The drawing under review shows one solid part. Ordinate dimensions are in mm from its lowest x, y, z. A direction names the side the tool comes from. Coordinates: 2 decimals unless noted, no trailing zeros. Write each loop counter-clockwise with the first axis right and the second up, starting at its lowest first coordinate (ties: lowest second). Pieces come first, ordered by that corner, then holes.
Q1. Take a section at C-C (z = 500). Give the boundary of the cut face in (x, y).
Q2. Insertion check: pin 1 (23 mm diameter, centred on x = 50, z = 500, fed in from +Y); pin 2 (1 mm diameter, centred on x = 314, y = 10.5, fed in from -Z); pin 3 (8 mm diameter, centred on y = 23.5, z = 164.5, fed in from -X); pin 4 (8 mm diameter, centred on y = 23.5, z = 101, fed in from +X). Each pin has a flat end and moves straight along its axis. Give the tip position at first contact, or say it passes through.
Q3. Machinability: for the marked faces 1 and 2, which of the approach directions +Z, -Z, +X, -X, +Y, -Y give a long, thin tool a straight path to every point of the face, cutting with its end or side? Answer none if there is none.
Q4. Take a section at D-D (x = 250). Give the boundary of the cut face in (y, z).
Q5. For probe 1 along X at (y, z) = (10.5, 500); probe 2 along Z at (x, y) = (450, 14.5); probe 3 along X at (y, z) = (27.5, 50), list the stretches that pass through material, from the lowest coordinate up.
Q6. Take a section at A-A (x = 450). Give the boundary of the cut face in (y, z), and give its area (3 significant figures).
Q7. Take a section at B-B (y = 24.5). Give the boundary of the cut face in (x, z).
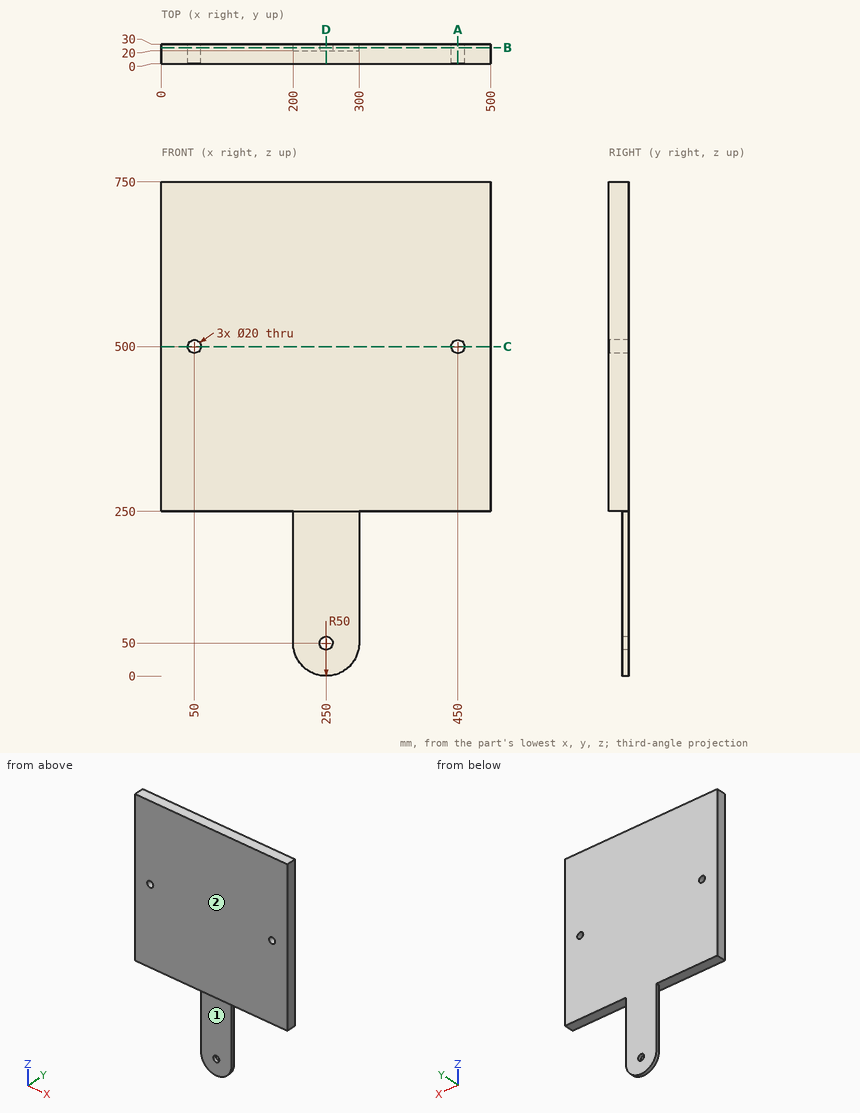
Response:
1. outline: (0, 0) - (40, 0) - (40, 30) - (0, 30) - close; (60, 0) - (440, 0) - (440, 30) - (60, 30) - close; (460, 0) - (500, 0) - (500, 30) - (460, 30) - close
2. pin 1: stops at y = 30
2. pin 2: stops at z = 250
2. pin 3: stops at x = 200
2. pin 4: stops at x = 300
3. face 1: -Z, +X, -X, -Y
3. face 2: +Z, -Z, +X, -X, -Y
4. outline: (0, 250) - (20, 250) - (20, 60) - (30, 60) - (30, 750) - (0, 750) - close; (20, 0) - (30, 0) - (30, 40) - (20, 40) - close
5. probe 1: x = 0 to 40, 60 to 440, 460 to 500
5. probe 2: z = 250 to 490, 510 to 750
5. probe 3: x = 200 to 240, 260 to 300
6. outline: (0, 250) - (30, 250) - (30, 490) - (0, 490) - close; (0, 510) - (30, 510) - (30, 750) - (0, 750) - close
6. area: 14,400 mm2
7. outline: (0, 250) - (200, 250) - (200, 50) arc R50 ccw to (300, 50) - (300, 250) - (500, 250) - (500, 750) - (0, 750) - close; hole circle Ø20 at (50, 500); hole circle Ø20 at (250, 50); hole circle Ø20 at (450, 500)
